```python
from build123d import *

# Parameters (mm, degrees)
F0_W     = 12.7625
F0_H     = 76.2625
F0_R     = 4
F0_R_2   = 1.35255
F0_W_2   = 8
F0_H_2   = 40.0949
F1_DEPTH = 6.35
F2_R     = 1.190625
F3_SIZE  = 0.254


with BuildPart() as f1:
    # F0 (on Top) → F1 (new body)
    with BuildSketch(Plane.XY):
        Rectangle(F0_W, F0_H)
        with Locations((0, -31.75)):
            Circle(F0_R, mode=Mode.SUBTRACT)
        with Locations((0, -24.0162)):
            Circle(F0_R_2, mode=Mode.SUBTRACT)
        Rectangle(F0_W_2, F0_H_2, mode=Mode.SUBTRACT)
        with Locations((0, 24.0162)):
            Circle(F0_R_2, mode=Mode.SUBTRACT)
        with Locations((0, 31.75)):
            Circle(F0_R, mode=Mode.SUBTRACT)
    extrude(amount=F1_DEPTH)

    # F2
    f2_edges = [f1.edges().sort_by_distance(p)[0] for p in [
        (-4, 20.04745, 3.175),
        (4, 20.04745, 3.175),
        (4, -20.04745, 3.175),
        (-4, -20.04745, 3.175),
    ]]
    fillet(f2_edges, radius=F2_R)

    # F3
    f3_edges = [f1.edges().sort_by_distance(p)[0] for p in [
        (-4, 31.75, 0),
        (-4, -31.75, 0),
    ]]
    chamfer(f3_edges, length=F3_SIZE)


solid = f1.part
```
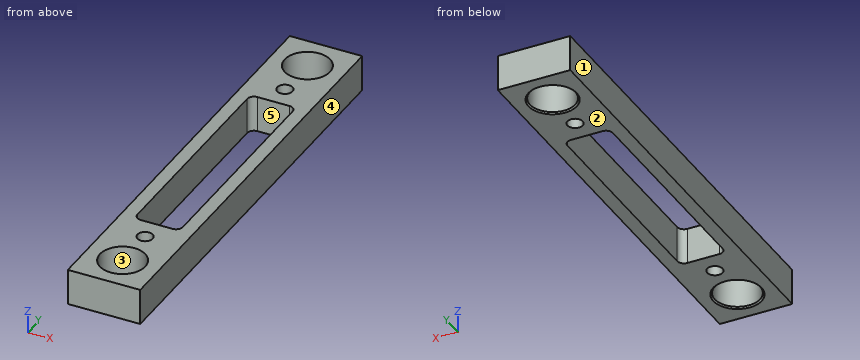
Build history of the part. All positions in model axes, mm. Face numbers are marked on the shaded views. A direction names the side the tool comes from. Give positions to 0.01 mm unless a question says otherwise; leave off trailing zeros. Order: outer loops, then holes, each group sorted by start corner. A loop starts at its lowest first (then second) coordinate and runs counter-clockwise, first axis right, second up. Notation, with made-up numbers: M 28.5,-27.5 L 46.5,-27.5 A19 cw 46.5,-4.5 Z; hole C 12.5,65 d8. An arc over 180 degrees is marked long. Write item = value, one per line. Start each with the question number.
(1) Slice it at B-B on x = 0. Write the cut outline in (y, z), plus the area to 3 significant figures.
(2) Slice it at D-D on y = 31.75. Write the cut outline in (x, z), plus the area to 3 significant figures.
(3) Probe L1, parallel to Y at x = 0, z = 4; L2, parallel to Y at x = 1.5, z = 4.75; L3, parallel to Y at x = -2.5, z = 5. List the from-to ranges inside material, lowest first. Write a range as [from, to].
(4) Which spindle directions (+Z, -Z, +X, -X, +Y, -Y) get a long thin tool onto all of the face, cutting with end or side? Do the marked faces 4 and 5. Say none if no direction does.
(5) Slice it at C-C on z = 1.5. Write the cut outline in (x, y).
(6) Slice it at A-A on y = 1.5. Write the cut outline in (x, z).
(7) Two-plate mould, pull along X, no slides. Class the marked faces 1, 2 and 3: released by +X, released by -X, zero draft, split by the parting line, or undercut.
Responses:
q1.outline = M -38.13,0 L -36,0 L -35.75,0.25 L -35.75,6.35 L -38.13,6.35 Z; M -27.75,0.25 L -27.5,0 L -25.37,0 L -25.37,6.35 L -27.75,6.35 Z; M -22.66,0 L -20.05,0 L -20.05,6.35 L -22.66,6.35 Z; M 20.05,0 L 22.66,0 L 22.66,6.35 L 20.05,6.35 Z; M 25.37,0 L 27.5,0 L 27.75,0.25 L 27.75,6.35 L 25.37,6.35 Z; M 35.75,0.25 L 36,0 L 38.13,0 L 38.13,6.35 L 35.75,6.35 Z
q1.area = 93.6 mm2
q2.outline = M -6.38,0 L -4.25,0 L -4,0.25 L -4,6.35 L -6.38,6.35 Z; M 4,0.25 L 4.25,0 L 6.38,0 L 6.38,6.35 L 4,6.35 Z
q2.area = 30.2 mm2
q3.L1 = [-38.13, -35.75], [-27.75, -25.37], [-22.66, -20.05], [20.05, 22.66], [25.37, 27.75], [35.75, 38.13]
q3.L2 = [-38.13, -35.46], [-28.04, -20.05], [20.05, 28.04], [35.46, 38.13]
q3.L3 = [-38.13, -34.87], [-28.63, -20.05], [20.05, 28.63], [34.87, 38.13]
q4.face_4 = +Z, -Z, +X, +Y, -Y
q4.face_5 = +Z, -Z
q5.outline = M -6.38,-38.13 L 6.38,-38.13 L 6.38,38.13 L -6.38,38.13 Z; hole C 0,-31.75 d8; hole M -4,-18.86 A1.19 ccw -2.81,-20.05 L 2.81,-20.05 A1.19 ccw 4,-18.86 L 4,18.86 A1.19 ccw 2.81,20.05 L -2.81,20.05 A1.19 ccw -4,18.86 Z; hole C 0,31.75 d8; hole C 0,-24.02 d2.71; hole C 0,24.02 d2.71
q6.outline = M -6.38,0 L -4,0 L -4,6.35 L -6.38,6.35 Z; M 4,0 L 6.38,0 L 6.38,6.35 L 4,6.35 Z
q7.face_1 = released by -X
q7.face_2 = zero draft
q7.face_3 = undercut
